Check sheet for the modelled part. Datum: model origin and axes. Units: mm. Face numbers are marked on the shaded views. A direction names the side the tool comes from. Give positions to 0.01 mm unless a question says otherwise; leave off trailing zeros. Loops run counter-clockwise (first coordinate to the right, second up) from the corner with the lowest first, then second, coordinate; pieces in that order, holes last. Notation, with made-up numbers: M 52.25,-3 L 74.25,-3 A6 cw 74.25,5 Z; hole C -15.75,5.25 d1. An arc over 180 degrees is marked long. Write each question's results on one line, items separated by ' | '. Start each with the question number.
1. Sectioned sample at C-C on x = 12. Record the cut outline in (y, z).
2. Tool access check on the marked faces 1 and 2. Record the directions out of +Z, -Z, +X, -X, +Y, -Y that give a thin tool (end or side, any length) a straight path to the whole face; none if there is none.
3. Draft check along X on the marked faces 3, 4 and 5. Enter one of: pulls with the +X half, pulls with the -X half, needs draft (parallel to the pull), parting line crosses it, or undercut.
4. Material ranges on line 1 along X through (y, z) = (45, 4.5); line 2 along Y through (x, z) = (19, 1.25); line 3 along Z through (x, y) = (42, 25.5), recorded low to high.
5. Sectioned sample at B-B on y = 20.5. Record the cut outline in (x, z).
6. Sectioned sample at A-A on z = 9.5. Record the cut outline in (x, y), and give its area (3 significant figures).
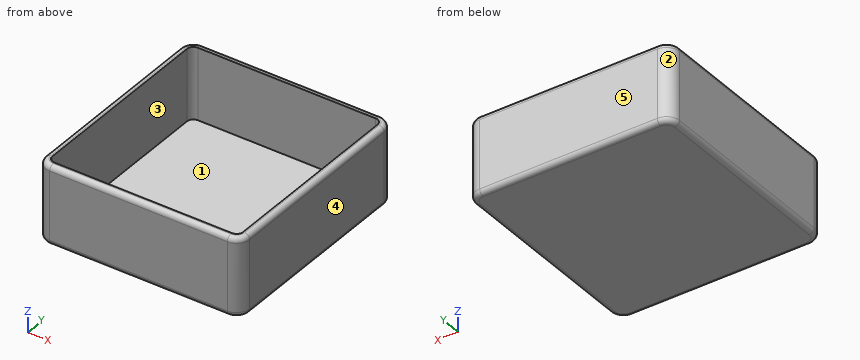
```python
from build123d import *

# Parameters (mm, degrees)
BOSS_EXTRU_1_DEPTH = 22
COQUE1_T           = 2
CONG_1_R           = 1.5
CONG_2_R           = 1.5


with BuildPart() as part:
    # Esquisse1 → Boss.-Extru.1 (new body)
    with BuildSketch(Plane.XY):
        with BuildLine():
            Line((2, 0), (56.5, 0))
            ThreePointArc((56.5, 0), (57.914213562, 0.585786438), (58.5, 2))
            Line((58.5, 2), (58.5, 60.5))
            ThreePointArc((58.5, 60.5), (57.914213562, 61.914213562), (56.5, 62.5))
            Line((56.5, 62.5), (2, 62.5))
            ThreePointArc((2, 62.5), (0.585786438, 61.914213562), (0, 60.5))
            Line((0, 60.5), (0, 2))
            ThreePointArc((0, 2), (0.585786438, 0.585786438), (2, 0))
        make_face()
    extrude(amount=BOSS_EXTRU_1_DEPTH)

    # Coque1
    coque1_openings = [part.faces().sort_by_distance(p)[0] for p in [
        (29.25, 31.25, 22),
    ]]
    offset(amount=COQUE1_T, openings=coque1_openings, kind=Kind.INTERSECTION)

    # Congé1
    # the kernel refuses this fillet: 1.5 mm, written as the material it takes off along each edge
    with BuildSketch(Plane(origin=(56.5, 60.5, 22), x_dir=(0, 1, 0), z_dir=(-1, 0, 0))) as cong_1_piece_1:
        with BuildLine():
            CenterArc((4 - CONG_1_R, CONG_1_R), CONG_1_R, 270, 90)
            Line((4, CONG_1_R), (4, 0))
            Line((4, 0), (4 - CONG_1_R, 0))
        make_face()
    revolve(axis=Axis((56.5, 60.5, 22), (0, 0, -1)), revolution_arc=90, mode=Mode.SUBTRACT)
    with BuildSketch(Plane(origin=(2, 64.5, 22), x_dir=(0, -1, 0), z_dir=(1, 0, 0)), Plane(origin=(56.5, -2, 22), x_dir=(0, 1, 0), z_dir=(-1, 0, 0))) as cong_1_piece_2:
        with BuildLine():
            CenterArc((CONG_1_R, CONG_1_R), CONG_1_R, 180, 90)
            Line((0, CONG_1_R), (0, 0))
            Line((0, 0), (CONG_1_R, 0))
        make_face()
    extrude(amount=54.5, mode=Mode.SUBTRACT)
    with BuildSketch(Plane(origin=(2, 60.5, 22), x_dir=(-1, 0, 0), z_dir=(0, -1, 0))) as cong_1_piece_3:
        with BuildLine():
            CenterArc((4 - CONG_1_R, CONG_1_R), CONG_1_R, 270, 90)
            Line((4, CONG_1_R), (4, 0))
            Line((4, 0), (4 - CONG_1_R, 0))
        make_face()
    revolve(axis=Axis((2, 60.5, 22), (0, 0, -1)), revolution_arc=90, mode=Mode.SUBTRACT)
    with BuildSketch(Plane(origin=(-2, 2, 22), x_dir=(1, 0, 0), z_dir=(0, 1, 0)), Plane(origin=(60.5, 60.5, 22), x_dir=(-1, 0, 0), z_dir=(0, -1, 0))) as cong_1_piece_4:
        with BuildLine():
            CenterArc((CONG_1_R, CONG_1_R), CONG_1_R, 180, 90)
            Line((0, CONG_1_R), (0, 0))
            Line((0, 0), (CONG_1_R, 0))
        make_face()
    extrude(amount=58.5, mode=Mode.SUBTRACT)
    with BuildSketch(Plane(origin=(2, 2, 22), x_dir=(0, -1, 0), z_dir=(1, 0, 0))) as cong_1_piece_5:
        with BuildLine():
            CenterArc((4 - CONG_1_R, CONG_1_R), CONG_1_R, 270, 90)
            Line((4, CONG_1_R), (4, 0))
            Line((4, 0), (4 - CONG_1_R, 0))
        make_face()
    revolve(axis=Axis((2, 2, 22), (0, 0, -1)), revolution_arc=90, mode=Mode.SUBTRACT)
    with BuildSketch(Plane(origin=(56.5, 2, 22), x_dir=(1, 0, 0), z_dir=(0, 1, 0))) as cong_1_piece_6:
        with BuildLine():
            CenterArc((4 - CONG_1_R, CONG_1_R), CONG_1_R, 270, 90)
            Line((4, CONG_1_R), (4, 0))
            Line((4, 0), (4 - CONG_1_R, 0))
        make_face()
    revolve(axis=Axis((56.5, 2, 22), (0, 0, -1)), revolution_arc=90, mode=Mode.SUBTRACT)

    # Congé2
    cong_2_edges = [part.edges().sort_by_distance(p)[0] for p in [
        (29.25, 64.5, -2),
        (59.328427125, 63.328427125, -2),
        (60.5, 31.25, -2),
        (59.328427125, -0.828427125, -2),
        (29.25, -2, -2),
        (-0.828427125, -0.828427125, -2),
        (-2, 31.25, -2),
        (-0.828427125, 63.328427125, -2),
    ]]
    fillet(cong_2_edges, radius=CONG_2_R)


solid = part.part
```
Output values:
1) outline: M -2,-0.5 A1.5 ccw -0.5,-2 L 63,-2 A1.5 ccw 64.5,-0.5 L 64.5,20.5 A1.5 ccw 63,22 L 62.5,22 L 62.5,0 L 0,0 L 0,22 L -0.5,22 A1.5 ccw -2,20.5 Z
2) face 1: +Z | face 2: +Z, -Z, -X, +Y
3) face 3: undercut | face 4: pulls with the +X half | face 5: needs draft
4) line 1: -2 to 0, 58.5 to 60.5 | line 2: -2 to 0, 62.5 to 64.5 | line 3: -2 to 0
5) outline: M -2,-0.5 A1.5 ccw -0.5,-2 L 59,-2 A1.5 ccw 60.5,-0.5 L 60.5,20.5 A1.5 ccw 59,22 L 58.5,22 L 58.5,0 L 0,0 L 0,22 L -0.5,22 A1.5 ccw -2,20.5 Z
6) outline: M -2,2 A4 ccw 2,-2 L 56.5,-2 A4 ccw 60.5,2 L 60.5,60.5 A4 ccw 56.5,64.5 L 2,64.5 A4 ccw -2,60.5 Z; hole M 0,2 A2 ccw 2,0 L 56.5,0 A2 ccw 58.5,2 L 58.5,60.5 A2 ccw 56.5,62.5 L 2,62.5 A2 ccw 0,60.5 Z | area: 490 mm2
